Design review of the part built by this model. Coordinates are the model's own, in mm. Coordinates: 2 decimals unless noted, no trailing zeros. Write each loop counter-clockwise with the first axis right and the second up, starting at its lowest first coordinate (ties: lowest second). Pieces come first, ordered by that corner, then holes.
Q1. Clearance check with flat-ended pins moving along their axes: pin 1 Ø4 at (x, z) = (62, -0.5) entering from -Y (3 decimals); pin 2 Ø23 at (x, y) = (-60.87, 19.78) entering from +Z; pin 3 Ø3 at (x, z) = (-56, 3.5) entering from -Y; pin 4 Ø2 at (x, z) = (17.5, -2.5) entering from +Y. State where each tip first meets the part, or that it passes through.
Q2. Add section A-A, the plane y = 0. Give the boundary of the cut face in (x, z).
Q3. Add section D-D, the plane x = -56. Give the boundary of the cut face in (y, z), plus the area to 3 significant figures.
Q4. Add section B-B, the plane x = 0. Give the boundary of the cut face in (y, z), plus the area to 4 significant figures.
Q5. To check wall thickness, follow probe 1 along Y at (x, z) = (0, 0.5); probe 2 along X at (y, z) = (-50, 0.25); probe 3 along Y at (x, z) = (-5, -1.75). State the ranges of each line that lie inside material, in increasing order.
Q6. The part is to be moulded in two halves that separate along Y. For faces 1 (the face through (17, 1, -5)), 2 (the face through (42.607, -57.038, 0.07)), 3 (the face through (-17.34, -78.1, 0.07)), say which applies: +Y half, -Y half, draft (parallel to the pull), parting line (faces both ways), or undercut.
Q7. Add section C-C, the plane z = 2.75. Give the boundary of the cut face in (x, y).
from build123d import *

# Parameters (mm, degrees)
ESQUISSE1_R                  = 80
ESQUISSE1_R_2                = 15
BOSS_EXTRU_1_DEPTH           = 5
ESQUISSE3_R                  = 7.25
ENL_V_MAT_EXTRU_1_DEPTH      = 10
R_P_TITION_CIRCULAIRE4_COUNT = 5


with BuildPart() as part:
    # Esquisse1 → Boss.-Extru.1 (new body, symmetric)
    with BuildSketch(Plane.XY):
        Circle(ESQUISSE1_R)
        Circle(ESQUISSE1_R_2, mode=Mode.SUBTRACT)
    extrude(amount=BOSS_EXTRU_1_DEPTH, both=True)

    # Esquisse3 → Enlèv. mat.-Extru.1 (cut)
    with BuildSketch(Plane.XY.offset(5)):
        with Locations((0, 64)):
            Circle(ESQUISSE3_R)
    enl_v_mat_extru_1 = extrude(amount=-ENL_V_MAT_EXTRU_1_DEPTH, mode=Mode.SUBTRACT)

    # Répétition circulaire4: Enlèv. mat.-Extru.1 ×5 about axis
    r_p_tition_circulaire4_axis = Axis((0, 0, 0), (0, 0, 1))
    for i in range(1, R_P_TITION_CIRCULAIRE4_COUNT):
        add(enl_v_mat_extru_1.rotate(r_p_tition_circulaire4_axis, i * 360 / R_P_TITION_CIRCULAIRE4_COUNT), mode=Mode.SUBTRACT)


solid = part.part
Here are the results:
1. pin 1: stops at y = -52.915
1. pin 2: stops at z = 5
1. pin 3: stops at y = -58.56
1. pin 4: stops at y = 78.28
2. outline: (-80, -5) - (-15, -5) - (-15, 5) - (-80, 5) - close; (15, -5) - (80, -5) - (80, 5) - (15, 5) - close
3. outline: (-57.13, -5) - (14.4, -5) - (14.4, 5) - (-57.13, 5) - close; (25.15, -5) - (57.13, -5) - (57.13, 5) - (25.15, 5) - close
3. area: 1,040 mm2
4. outline: (-80, -5) - (-15, -5) - (-15, 5) - (-80, 5) - close; (15, -5) - (56.75, -5) - (56.75, 5) - (15, 5) - close; (71.25, -5) - (80, -5) - (80, 5) - (71.25, 5) - close
4. area: 1,155 mm2
5. probe 1: y = -80 to -15, 15 to 56.75, 71.25 to 80
5. probe 2: x = -62.45 to -44.65, -30.59 to 30.59, 44.65 to 62.45
5. probe 3: y = -79.84 to -14.14, 14.14 to 58.75, 69.25 to 79.84
6. face 1: draft
6. face 2: undercut
6. face 3: parting line
7. outline: circle Ø160 at (0, 0); hole circle Ø14.5 at (-60.87, 19.78); hole circle Ø14.5 at (-37.62, -51.78); hole circle Ø30 at (0, 0); hole circle Ø14.5 at (0, 64); hole circle Ø14.5 at (37.62, -51.78); hole circle Ø14.5 at (60.87, 19.78)
